Read the model definition and answer for the solid it produces. Units are mm, in the model's axes. Coordinates: 2 decimals unless noted, no trailing zeros. Order: outer loops, then holes, each group sorted by start corner. A loop starts at its lowest first (then second) coordinate and runs counter-clockwise, first axis right, second up. Notation, with made-up numbers: (88.5, 82) -> (122.5, 82) arc R25 cw to (122.5, 100) -> close; hole circle Ø4 at (83.5, 7.5). An arc over 180 degrees is marked (long way). Answer as a JSON object with one key per item and string values. Group by question number.
1) Section A-A on z = 0 is taken. Determine the outline of the cut face in (x, y), and give its area (3 significant figures).
2) Section C-C on x = 76 is taken. Determine the outline of the cut face in (y, z).
3) Section B-B on x = 41 is taken. Determine the outline of the cut face in (y, z), and give its area (3 significant figures).
4) Consider L1, parallel to Z at x = 85.5, y = -0.75; L2, parallel to Y at x = 115, z = -4.4. Determine where each line is inside the solid, lowest interval first.
5) Section D-D on y = 0 is taken. Count the separate pieces of the cut face and the enclosed holes in it, and give its area (3 significant figures).
from build123d import *

# Parameters (mm, degrees)
SKETCH_1_W          = 10
SKETCH_1_H          = 10
SKETCH_1_W_2        = 8
SKETCH_1_H_2        = 8
EXTRUDE_1_DEPTH     = 120
SKETCH_2_R          = 2
CUT_EXTRUDE_1_DEPTH = 121.519707932
SKETCH_3_R          = 1.5
CUT_EXTRUDE_2_DEPTH = 121.519707932


with BuildPart() as part:
    # ｽｹｯﾁ1 → 押し出し-薄板1 (new body)
    with BuildSketch(Plane(origin=(0, 0, 0), x_dir=(0, 0, -1), z_dir=(1, 0, 0))):
        Rectangle(SKETCH_1_W, SKETCH_1_H)
        Rectangle(SKETCH_1_W_2, SKETCH_1_H_2, mode=Mode.SUBTRACT)
    extrude(amount=EXTRUDE_1_DEPTH)

    # ｽｹｯﾁ2 → ｶｯﾄ - 押し出し1 (cut, through all)
    with BuildSketch(Plane(origin=(0, 5, 0), x_dir=(1, 0, 0), z_dir=(0, 1, 0))):
        with Locations(Location((44, 0, 0), (0, 0, 270))):
            Circle(SKETCH_2_R)
        with Locations(Location((76, 0, 0), (0, 0, 270))):
            Circle(SKETCH_2_R)
    extrude(amount=-CUT_EXTRUDE_1_DEPTH, mode=Mode.SUBTRACT)

    # ｽｹｯﾁ3 → ｶｯﾄ - 押し出し2 (cut, through all)
    with BuildSketch(Plane.XY.offset(5)):
        with Locations((5, 0)):
            Circle(SKETCH_3_R)
        with Locations(Location((115, 0, 0), (0, 0, 180))):
            Circle(SKETCH_3_R)
        with Locations((25, 0)):
            Circle(SKETCH_3_R)
        with Locations(Location((95, 0, 0), (0, 0, 180))):
            Circle(SKETCH_3_R)
    extrude(amount=-CUT_EXTRUDE_2_DEPTH, mode=Mode.SUBTRACT)


solid = part.part
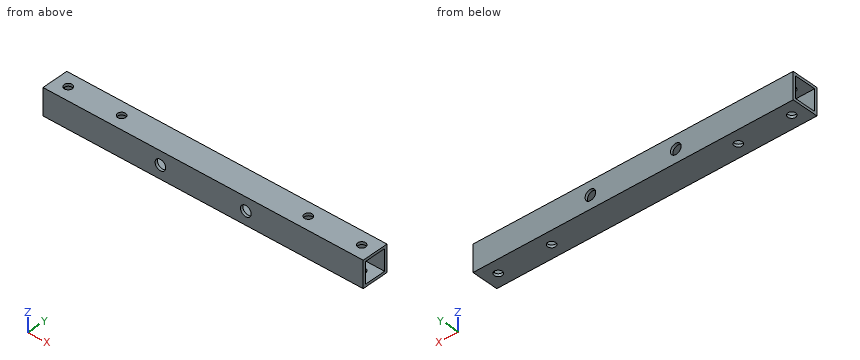
Worked answers:
{
 "1": {"outline": "(0, -5) -> (42, -5) -> (42, -4) -> (0, -4) -> close; (0, 4) -> (42, 4) -> (42, 5) -> (0, 5) -> close; (46, -5) -> (74, -5) -> (74, -4) -> (46, -4) -> close; (46, 4) -> (74, 4) -> (74, 5) -> (46, 5) -> close; (78, -5) -> (120, -5) -> (120, -4) -> (78, -4) -> close; (78, 4) -> (120, 4) -> (120, 5) -> (78, 5) -> close", "area": "224 mm²"},
 "2": {"outline": "(-5, -5) -> (5, -5) -> (5, -2) -> (4, -2) -> (4, -4) -> (-4, -4) -> (-4, -2) -> (-5, -2) -> close; (-5, 2) -> (-4, 2) -> (-4, 4) -> (4, 4) -> (4, 2) -> (5, 2) -> (5, 5) -> (-5, 5) -> close"},
 "3": {"outline": "(-5, -5) -> (5, -5) -> (5, 5) -> (-5, 5) -> close; hole (-4, -4) -> (4, -4) -> (4, 4) -> (-4, 4) -> close", "area": "36.0 mm²"},
 "4": {"L1": "z = -5 to -4, 4 to 5", "L2": "y = -5 to -1.5, 1.5 to 5"},
 "5": {"separate pieces": "10", "enclosed holes": "0", "area": "216 mm²"}
}
